Work out the finished part from the listing and answer in its coordinate system (mm). A direction names the side the tool comes from. Coordinates: 2 decimals unless noted, no trailing zeros. Loops run counter-clockwise (first coordinate to the right, second up) from the corner with the lowest first, then second, coordinate; pieces in that order, holes last.
```python
from build123d import *

# Parameters (mm, degrees)
F0_W       = 101.6
F0_H       = 101.6
F1_DEPTH   = 101.6
F2_R       = 25.4
F1_FACE_W  = 50.8
F1_FACE_H  = 50.8
F1_FACE1_W = 50.8
F1_FACE1_H = 50.8
F1_FACE2_W = 50.8
F1_FACE2_H = 50.8


with BuildPart() as f1:
    # F0 (on Top) → F1 (new body)
    with BuildSketch(Plane.XY):
        Rectangle(F0_W, F0_H)
    extrude(amount=F1_DEPTH)

    # F2
    f2_edges = [f1.edges().sort_by_distance(p)[0] for p in [
        (50.8, 0, 101.6),
        (0, -50.8, 101.6),
        (-50.8, 0, 101.6),
        (0, 50.8, 101.6),
        (50.8, 50.8, 50.8),
        (50.8, -50.8, 50.8),
        (-50.8, -50.8, 50.8),
        (0, -50.8, 0),
        (50.8, 0, 0),
        (0, 50.8, 0),
        (-50.8, 50.8, 50.8),
        (-50.8, 0, 0),
    ]]
    fillet(f2_edges, radius=F2_R)

    # F1_face (on face) → F3 (revolve)
    with BuildSketch(Plane.XY.offset(101.6)):
        Rectangle(F1_FACE_W, F1_FACE_H)
    revolve(axis=Axis((-50.8, -25.4, 76.2), (1, 0, 0)))

    # F1_face1 (on face) → F4 (revolve)
    with BuildSketch(Plane(origin=(0, 50.8, 50.8), x_dir=(-1, 0, 0), z_dir=(0, 1, 0))):
        Rectangle(F1_FACE1_W, F1_FACE1_H)
    revolve(axis=Axis((25.4, 25.4, 0), (0, 0, 1)))

    # F1_face2 (on face) → F5 (revolve)
    with BuildSketch(Plane(origin=(-50.8, 0, 50.8), x_dir=(0, -1, 0), z_dir=(-1, 0, 0))):
        Rectangle(F1_FACE2_W, F1_FACE2_H)
    revolve(axis=Axis((-25.4, 50.8, 25.4), (0, -1, 0)))


solid = f1.part
```
1. A cutting plane is placed at C-C, the plane x = -62.5. Give the vertices of the cut face in (y, z), then the cut area to 3 significant figures.
2. A cutting plane is placed at B-B, the plane y = -4. Give the vertices of the cut face in (x, z), then the cut area to 3 significant figures.
3. For faces 1 (the flat face through (25.4, -53, 92)), 2 (the flat face through (40, 53, 25.4)), 3 (the flat face through (-41, -25.4, -2)), 4 (the flat face through (40, 53, 76.2)), determine the directions among +Z, -Z, +X, -X, +Y, -Y from which every point of the face is accessible in a straight line to the end or side of a thin tool.
4. Each of these flat-tipped pins is pushed along its axis until it touches: P1, Ø8, axis at y = -51.5, z = 104, coming from the +X side; P2, Ø8, axis at y = 1.5, z = 48.5, coming from the -X side; P3, Ø8, axis at x = 38.5, y = -31.5, coming from the -Z side. Where does it stop, or does it pass through?
5. A cutting plane is placed at D-D, the plane z = -21. Give the vertices of the cut face in (x, y), then the cut area to 3 significant figures.
6. Straight lines are drawn through the part: probe 1 along X at (y, z) = (-23, 107.5); probe 2 along Z at (x, y) = (-3, 55.5). For each, find the intervals that lie inside material, in ascending order.
7. A cutting plane is placed at A-A, the plane z = 86. Give the vertices of the cut face in (x, y), then the cut area to 3 significant figures.
Answers below:
1. outline: (-25.4, -17.6) - (25.4, -17.6) - (25.4, 68.4) - (-25.4, 68.4) - close
1. area: 4,370 mm2
2. outline: (-50.8, 76.2) arc R56.8 ccw (long way) to (25.4, 0) arc R25.4 ccw to (50.8, 25.4) - (73.99, 25.4) - (73.99, 76.2) - (50.8, 76.2) arc R25.4 ccw to (25.4, 101.6) - (25.4, 128.81) - (-25.4, 128.81) - (-25.4, 101.6) arc R25.4 ccw to start
2. area: 16,600 mm2
3. face 1: +Z, +X, -Y
3. face 2: -Z, +X, +Y
3. face 3: -Z, -X, -Y
3. face 4: +Z, +X, +Y
4. P1: stops at x = 25.4
4. P2: stops at x = -78.89
4. P3: stops at z = 2.25
5. outline: (-58.15, -25.4) - (7.35, -25.4) - (7.35, 25.4) - (-58.15, 25.4) - close
5. area: 3,330 mm2
6. probe 1: x = -25.4 to 25.4
6. probe 2: z = 25.4 to 76.2
7. outline: (-48.83, -25.4) arc R23.43 ccw to (-25.4, -48.83) - (-25.4, -81.34) - (25.4, -81.34) - (25.4, -48.83) arc R23.43 ccw to (48.83, -25.4) - (48.83, 25.4) arc R23.43 ccw to (25.4, 48.83) - (-25.4, 48.83) arc R23.43 ccw to (-48.83, 25.4) - close
7. area: 10,700 mm2
